Drawing for the job (mm, zero at the part's lowest x, y, z). A direction names the side the tool comes from. Give positions to 0.01 mm unless a question says otherwise; leave off trailing zeros. Write each loop counter-clockwise with the first axis right and the second up, starting at its lowest first coordinate (ties: lowest second). Pieces come first, ordered by that corner, then holes. Notation, with made-up numbers: (74, -14.5) - (81, -14.5) arc R23 ccw to (81, 17.5) - close; hole circle Ø7 at (-37.75, 19). An arc over 180 degrees is marked (long way). Use CSV: the item, a comma, the result in double quotes.
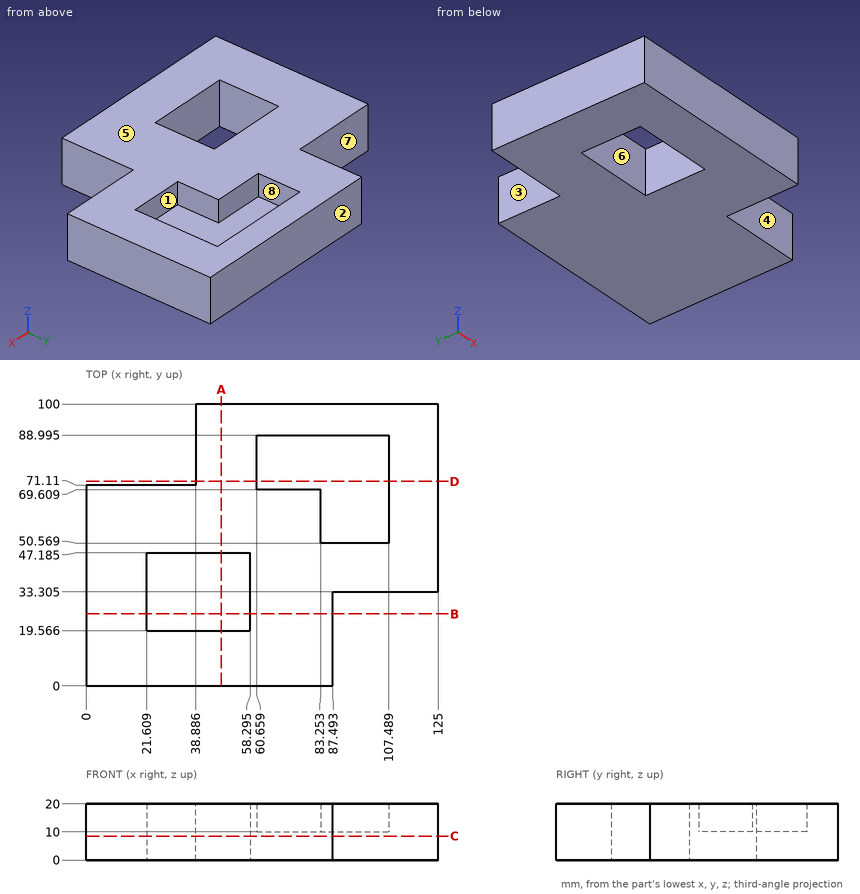
(1) Saw through at A-A, the plane x = 48. List the corners of the cut face in (y, z) (1 decimal).
Checked values:
outline,"(0, 0) - (19.6, 0) - (19.6, 20) - (0, 20) - close; (47.2, 0) - (100, 0) - (100, 20) - (47.2, 20) - close"
(2) Saw through at D-D, the plane y = 72.5. List the corners of the cut face in (x, z) (1 decimal).
Checked values:
outline,"(38.9, 0) - (125, 0) - (125, 20) - (107.5, 20) - (107.5, 10) - (60.7, 10) - (60.7, 20) - (38.9, 20) - close"
(3) Saw through at C-C, the plane z = 8.5. List the corners of the cut face in (x, y) (1 decimal).
Checked values:
outline,"(0, 0) - (87.5, 0) - (87.5, 33.3) - (125, 33.3) - (125, 100) - (38.9, 100) - (38.9, 71.1) - (0, 71.1) - close; hole (21.6, 19.6) - (58.3, 19.6) - (58.3, 47.2) - (21.6, 47.2) - close"
(4) Flat gauge pins, fed straight in: P1, Ø10, axis at x = 114.5, z = 13, coming from the -Y side (1 decimal); P2, Ø5, axis at x = 48.5, y = 45, coming from the +Z side; P3, Ø6, axis at y = 80, z = 5.5, coming from the -X side; P4, Ø5, axis at x = 86, y = 77.5, coming from the +Z side. Where does each tip first touch, or does it go through?
Checked values:
P1,"stops at y = 33.3"
P2,"stops at z = 20"
P3,"stops at x = 38.89"
P4,"stops at z = 10"
(5) Pull direction Y, two halves, no side cores. Call the marked faces 1, 2, 3 and 4: released by +Y, released by -Y, zero draft, split by the parting line, or undercut.
Checked values:
face 1,"undercut"
face 2,"released by +Y"
face 3,"zero draft"
face 4,"released by -Y"
(6) 3-axis set-ups, long thin cutter, end or side, ignore diameter. For the marked faces 5, 6, 7 and 8: which of +Z, -Z, +X, -X, +Y, -Y reach the whole face in a straight line?
Checked values:
face 5,"+Z, +X, -X, +Y, -Y"
face 6,"+Z, -Z"
face 7,"+Z, -Z, -X, +Y"
face 8,"+Z"
(7) Saw through at B-B, the plane y = 25.5. List the corners of the cut face in (x, z) (1 decimal).
Checked values:
outline,"(0, 0) - (21.6, 0) - (21.6, 20) - (0, 20) - close; (58.3, 0) - (87.5, 0) - (87.5, 20) - (58.3, 20) - close"
(8) Wall check: probe 1 along Y at (x, z) = (45.5, 17.5) (1 decimal); probe 2 along X at (y, z) = (26.5, 14) (1 decimal); probe 3 along Y at (x, z) = (28.5, 8.25) (1 decimal). Give the ranges that are in metal, low to high. Write a range as [from, to].
Checked values:
probe 1,"y = [0, 19.6], [47.2, 100]"
probe 2,"x = [0, 21.6], [58.3, 87.5]"
probe 3,"y = [0, 19.6], [47.2, 71.1]"
